Autodesk Inventor part; units mm, degrees
ref_plane "YZ Plane" through (0, 0, 0) normal (1, 0, 0) x (0, 1, 0)
ref_plane "XZ Plane" through (0, 0, 0) normal (0, 1, 0) x (-1, 0, 0)
ref_plane "XY Plane" through (0, 0, 0) normal (0, 0, 1) x (1, 0, 0)
sketch "Sketch1" plane through (0, 0, 0) normal (0, 1, 0) x (-1, 0, 0)
  line L0 (0, 0) -> (-100, 0)
  line L1 (-100, 0) -> (-100, -42)
  line L2 (-100, -42) -> (0, -42)
  line L3 (0, -42) -> (0, 0)
  dimension "d0" = 100
  dimension "d1" = 42
extrude "Extrusion1" add sketch "Sketch1" along normal blind 4
sketch "Sketch2" plane through (0, 4, 0) normal (0, 1, 0) x (1, 0, 0)
  line L0 (0, 0) -> (100, 0) construction
  line L1 (100, 0) -> (100, 42) construction
  line L2 (100, 42) -> (0, 42) construction
  line L3 (0, 42) -> (0, 0) construction
  line L4 (4, 38) -> (96, 38) construction
  line L5 (96, 38) -> (96, 4) construction
  line L6 (96, 4) -> (4, 4) construction
  line L7 (4, 4) -> (4, 38) construction
  line L8 (100, 42) -> (0, 42)
  line L9 (4, 42) -> (4, 34)
  line L10 (4, 34) -> (0, 34)
  line L11 (0, 42) -> (0, 0)
  line L12 (0, 34) -> (0, 42)
  line L13 (0, 42) -> (4, 42)
  line L14 (0, 21) -> (100, 21) construction
  line L15 (50, 42) -> (50, 0) construction
  line L16 (0, 0) -> (100, 0) construction
  line L17 (0, 21) -> (0, 25)
  line L18 (4, 25) -> (0, 25)
  line L19 (4, 25) -> (4, 21)
  line L20 (14, 42) -> (14, 38)
  line L21 (14, 38) -> (22, 38)
  line L22 (22, 38) -> (22, 42)
  line L23 (14, 42) -> (22, 42)
  line L24 (30, 42) -> (38, 42)
  line L25 (38, 42) -> (38, 38)
  line L26 (38, 38) -> (30, 38)
  line L27 (30, 38) -> (30, 42)
  line L28 (50, 38) -> (46, 38)
  line L29 (46, 38) -> (46, 42)
  line L30 (46, 42) -> (50, 42)
  line L31 (4, 0) -> (4, 8)
  line L32 (4, 8) -> (0, 8)
  line L33 (0, 8) -> (0, 0)
  line L34 (0, 0) -> (4, 0)
  line L35 (0, 21) -> (0, 17)
  line L36 (4, 17) -> (0, 17)
  line L37 (4, 17) -> (4, 21)
  line L38 (14, 0) -> (14, 4)
  line L39 (14, 4) -> (22, 4)
  line L40 (22, 4) -> (22, 0)
  line L41 (14, 0) -> (22, 0)
  line L42 (30, 0) -> (38, 0)
  line L43 (38, 0) -> (38, 4)
  line L44 (38, 4) -> (30, 4)
  line L45 (30, 4) -> (30, 0)
  line L46 (50, 4) -> (46, 4)
  line L47 (46, 4) -> (46, 0)
  line L48 (46, 0) -> (50, 0)
  line L49 (100, 42) -> (100, 0) construction
  line L50 (96, 4) -> (96, 38) construction
  line L51 (96, 42) -> (96, 34)
  line L52 (96, 34) -> (100, 34)
  line L53 (100, 42) -> (100, 0)
  line L54 (100, 34) -> (100, 42)
  line L55 (100, 42) -> (96, 42)
  line L56 (100, 21) -> (100, 25)
  line L57 (96, 25) -> (100, 25)
  line L58 (96, 25) -> (96, 21)
  line L59 (86, 42) -> (86, 38)
  line L60 (86, 38) -> (78, 38)
  line L61 (78, 38) -> (78, 42)
  line L62 (86, 42) -> (78, 42)
  line L63 (70, 42) -> (62, 42)
  line L64 (62, 42) -> (62, 38)
  line L65 (62, 38) -> (70, 38)
  line L66 (70, 38) -> (70, 42)
  line L67 (50, 38) -> (54, 38)
  line L68 (54, 38) -> (54, 42)
  line L69 (54, 42) -> (50, 42)
  line L70 (70, 4) -> (70, 0)
  line L71 (62, 4) -> (70, 4)
  line L72 (70, 0) -> (62, 0)
  line L73 (62, 0) -> (62, 4)
  line L74 (54, 4) -> (54, 0)
  line L75 (50, 4) -> (54, 4)
  line L76 (54, 0) -> (50, 0)
  line L77 (78, 4) -> (78, 0)
  line L78 (86, 4) -> (78, 4)
  line L79 (86, 0) -> (78, 0)
  line L80 (86, 0) -> (86, 4)
  line L81 (96, 0) -> (96, 8)
  line L82 (100, 0) -> (96, 0)
  line L83 (96, 8) -> (100, 8)
  line L84 (100, 8) -> (100, 0)
  line L85 (96, 17) -> (96, 21)
  line L86 (100, 21) -> (100, 17)
  line L87 (96, 17) -> (100, 17)
  dimension "d4" = 4
  dimension "d5" = 4
  dimension "d7" = 8
  dimension "d8" = 8
  dimension "d10" = 8
  dimension "d11" = 8
  dimension "d13" = 4
  dimension "d14" = 8
extrude "Extrusion2" cut sketch "Sketch2" against normal up to surface (4 mm away)
sketch "Sketch3" plane through (0, 4, 0) normal (0, 1, 0) x (1, 0, 0)
  line L0 (4, 25) -> (4, 17)
  line L1 (96, 0) -> (96, 8)
  line L2 (4, 20) -> (96, 20)
  line L3 (96, 20) -> (96, 12)
  line L4 (96, 12) -> (4, 12)
  line L5 (4, 12) -> (4, 20)
  line L6 (30, 4) -> (38, 4)
  point P0 (0, 0)
  dimension "d17" = 8
  dimension "d18" = 8
extrude "Extrusion3" add sketch "Sketch3" along normal blind 3
properties part number "front" material "PBT Plastic Black"
Can you work these out from the model? Positions are in its coordinate system, mm. A direction names the side the tool comes from. Give positions to 0.01 mm unless a question says otherwise; leave off trailing zeros. Loops run counter-clockwise (first coordinate to the right, second up) from the corner with the lowest first, then second, coordinate; pieces in that order, holes last. Notation, with made-up numbers: M 54.25,79 L 83.25,79 A37 ccw 83.25,116 Z; hole C 57,55 d10. An arc over 180 degrees is marked long. Answer in a Markdown table with one row per item.
1. Suppose I cut it at A-A on x = 31.5. Write out the boundary of the cut face in (y, z).
Taken from the geometry:
| item | result |
|---|---|
| outline | M 0,-38 L 4,-38 L 4,-20 L 7,-20 L 7,-12 L 4,-12 L 4,-4 L 0,-4 Z |
2. If I drill on line 1 along Y through (x, z) = (37, -7.5); line 2 along X through (y, z) = (4.75, -16); line 3 along Z through (x, y) = (37, 3.5), over which ranges is the centre line in solid material (lowest first)?
Taken from the geometry:
| item | result |
|---|---|
| line 1 | y = 0 to 4 |
| line 2 | x = 4 to 96 |
| line 3 | z = -38 to -4 |
3. Suppose I cut it at D-D on z = -23. Write out the boundary of the cut face in (x, y).
Taken from the geometry:
| item | result |
|---|---|
| outline | M 4,0 L 96,0 L 96,4 L 4,4 Z |
4. For pin 1 Ø1.5 at (y, z) = (2.5, -20) entering from -X; pin 2 Ø4 at (x, z) = (86.5, -36) entering from -Y; pin 3 Ø1.2 at (y, z) = (2, -1.5) entering from +X; pin 4 Ø3 at (x, y) = (98, 2.5) entering from -Z, each with a flat end and sliding along its axis, tell me the tip position at first contact or that it passes through.
Taken from the geometry:
| item | result |
|---|---|
| pin 1 | stops at x = 4 |
| pin 2 | stops at y = 0 |
| pin 3 | stops at x = 96 |
| pin 4 | stops at z = -34 |
5. Suppose I cut it at C-C on y = 5.75. Write out the boundary of the cut face in (x, z).
Taken from the geometry:
| item | result |
|---|---|
| outline | M 4,-20 L 96,-20 L 96,-12 L 4,-12 Z |
6. Thinking about a two-plate mould opening in Z: for faces 1 (the flat face through (58, 2, 0)), 2 (the flat face through (96, 3, -19)), 3 (the flat face through (100, 2, -12)), which applies, released by +Z, released by -Z, zero draft, split by the parting line, or undercut?
Taken from the geometry:
| item | result |
|---|---|
| face 1 | released by +Z |
| face 2 | undercut |
| face 3 | zero draft |
7. Which directions (+Z, -Z, +X, -X, +Y, -Y) give clear straight access to the entire face, cutting with the end or side of a thin tool? Please do faces 4 (the flat face through (70, 2, -2)), 5 (the flat face through (4, 2, -4)), 6 (the flat face through (70, 2, -40)), 7 (the flat face through (49, 5, -20)).
Taken from the geometry:
| item | result |
|---|---|
| face 4 | +Z, +Y, -Y |
| face 5 | +Z, -X, +Y, -Y |
| face 6 | -Z, +Y, -Y |
| face 7 | -Z, +X, -X, +Y |
8. Suppose I cut it at B-B on z = -15. Write out the boundary of the cut face in (x, y).
Taken from the geometry:
| item | result |
|---|---|
| outline | M 0,0 L 100,0 L 100,4 L 96,4 L 96,7 L 4,7 L 4,4 L 0,4 Z |
